Job drawing, mm, ordinate dimensions from the low corner. One solid piece. A direction names the side the tool comes from. Give positions to 0.01 mm unless a question says otherwise; leave off trailing zeros. Order: outer loops, then holes, each group sorted by start corner. A loop starts at its lowest first (then second) coordinate and runs counter-clockwise, first axis right, second up. Notation, with made-up numbers: (-30, 86.5) - (19, 86.5) arc R16 cw to (19, 97.5) - close; hole circle Ø10 at (88, 34.25). An arc over 180 degrees is marked (long way). Use one line per item in the form item = value. Start each with the question number.
1. Drill centre lines: line 1 (Y direction, x = 2.1, z = 3.75); line 2 (Z direction, x = 2, y = 2.75). Where is each one in solid material? Low to high.
2. Pin check, flat tips, straight feed: P1, Ø0.5, axis at y = 2, z = 0, coming from the -X side; P2, Ø0.5, axis at x = 1.5, z = 0, coming from the +Y side; P3, Ø1, axis at x = 2.5, z = 4.5, coming from the +Y side. Stop position of each tip, or through.
3. Tool access for the marked faces 1 and 2: list every direction of +Z, -Z, +X, -X, +Y, -Y with a clear straight run to the whole face (end or side of a thin tool).
4. Band-saw the part on A-A, the plane z = 8.5. List the corners of the cut face in (x, y).
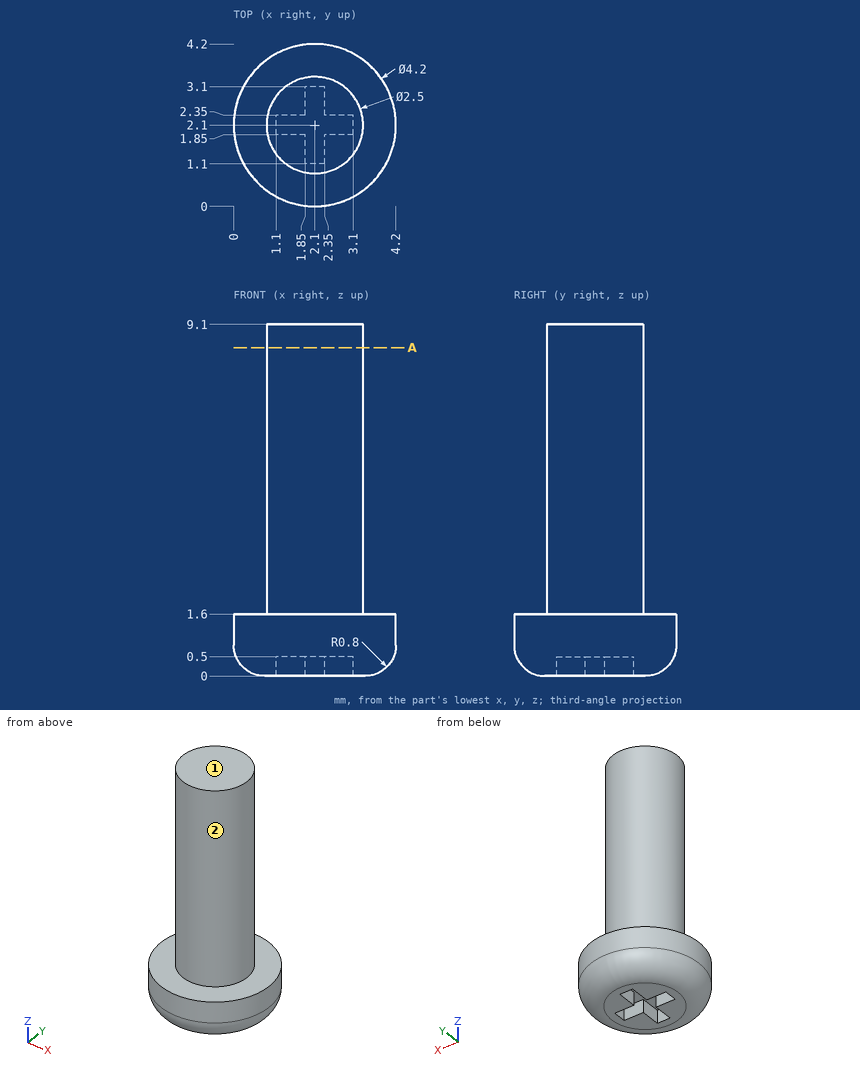
From the geometry:
q1.line_1 = 0.85 to 3.35
q1.line_2 = 0.5 to 9.1
q2.P1 = 0.22
q2.P2 = 3.89
q2.P3 = 3.35
q3.face_1 = +Z, +X, -X, +Y, -Y
q3.face_2 = +Z
q4.outline = circle Ø2.5 at (2.1, 2.1)
